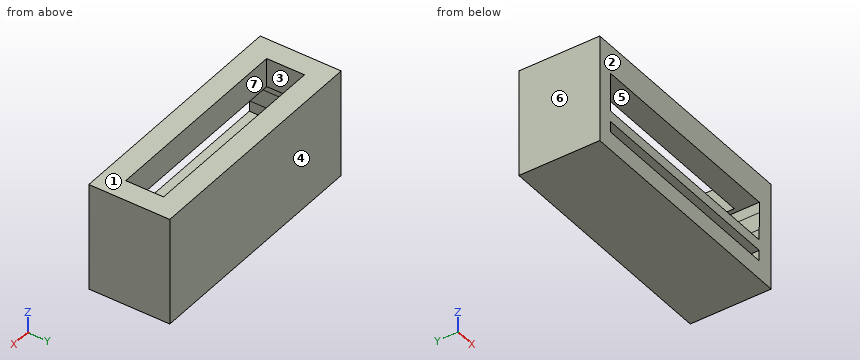
```python
from build123d import *

# Parameters (mm, degrees)
F0_W     = 114.3
F0_H     = 38.1
F1_DEPTH = 50.8
F2_W     = 93.98
F2_H     = 17.78
F3_DEPTH = 38.1
F4_W     = 99.06
F4_H     = 5.08
F5_DEPTH = 25.4
F6_DEPTH = 25.4


# Not quite as in the source:
# - a feature names something its author has since deleted; it is built from what else it names


with BuildPart() as f1:
    # F0 (on Top) → F1 (new body)
    with BuildSketch(Plane.XY):
        with Locations((-0.8744271472, -29.0754930802)):
            Rectangle(F0_W, F0_H)
    extrude(amount=F1_DEPTH)

    # F2 (on face) → F3 (cut)
    with BuildSketch(Plane.XY.offset(50.8)):
        with Locations((-0.8926133716, -29.0383800721)):
            Rectangle(F2_W, F2_H)
    extrude(amount=-F3_DEPTH, mode=Mode.SUBTRACT)

    # F4 (on face) → F5 (cut)
    with BuildSketch(Plane.XZ.offset(48.1254930802)):
        with Locations((-1.2216676867, 11.2467280274)):
            Rectangle(F4_W, F4_H)
        Polygon((-50.7150366902, 32.0992726219), (-50.7516676867, 23.9467280274), (48.3083323133, 23.9467280274), (48.3449633098, 32.0992726219), align=None)
        with Locations((-1.2216676867, 21.4067280274)):
            Rectangle(F4_W, F4_H)
        with Locations((-1.1850366902, 34.6392726219)):
            Rectangle(F4_W, F4_H)
    extrude(amount=-F5_DEPTH, mode=Mode.SUBTRACT)

    # F4 (on face) → F6 (cut)
    with BuildSketch(Plane.XZ.offset(48.1254930802)):
        with Locations((-1.2216676867, 11.2467280274)):
            Rectangle(F4_W, F4_H)
        Polygon((-50.7150366902, 32.0992726219), (-50.7516676867, 23.9467280274), (48.3083323133, 23.9467280274), (48.3449633098, 32.0992726219), align=None)
        with Locations((-1.2216676867, 21.4067280274)):
            Rectangle(F4_W, F4_H)
        with Locations((-1.1850366902, 34.6392726219)):
            Rectangle(F4_W, F4_H)
    extrude(amount=-F6_DEPTH, mode=Mode.SUBTRACT)


solid = f1.part
```
Read the model definition and answer for the solid it produces. Units are mm, in the model's axes. Face numbers are marked on the shaded views. A direction names the side the tool comes from. Coordinates: 2 decimals unless noted, no trailing zeros. Write each loop counter-clockwise with the first axis right and the second up, starting at its lowest first coordinate (ties: lowest second). Pieces come first, ordered by that corner, then holes. Notation, with made-up numbers: (49, 55) - (67, 55) arc R6 ccw to (67, 64) - close; hole circle Ø10 at (-15, -15.75). An arc over 180 degrees is marked (long way). Answer as a JSON object with one key per item and string values. Group by question number.
1. Which of the six approach directions +Z, -Z, +X, -X, +Y, -Y give full straight-line access (tool end or side, diameter ignored) to the marked faces 5, 6 and 7?
2. A cutting plane is placed at C-C (x = -32). Determine the outline of the cut face in (y, z), plus the area to 3 significant figures.
3. The mould has two halves that part along Y. Classify the marked faces 1, 2, 3 and 4: +Y half, -Y half, draft (parallel to the pull), parting line (faces both ways), or undercut.
4. Consider L1, parallel to Z at x = 14, y = -41; L2, parallel to X at y = -29, z = 49.5; L3, parallel to X at y = -28.5, z = 37. Determine where each line is inside the solid, lowest interval first. Write a range as [from, to].
5. Each of these flat-tipped pins is pushed along its axis until it touches: P1, Ø1.3, axis at x = 8, y = -21, coming from the +Z side; P2, Ø2.5, axis at x = -26, z = 12, coming from the -Y side; P3, Ø12.5, axis at x = -22.5, y = -29.5, coming from the +Z side. Where does it stop, or does it pass through?
6. A cutting plane is placed at B-B (y = -43.5). Determine the outline of the cut face in (x, z).
7. A cutting plane is placed at A-A (z = 42). Determine the outline of the cut face in (x, y).
8. A cutting plane is placed at D-D (y = -24.5). Determine the outline of the cut face in (x, z).
Worked out:
{
 "1": {"face 5": "-Y", "face 6": "+Z, -Z, -X, +Y, -Y", "face 7": "+Z"},
 "2": {"outline": "(-48.13, 0) - (-10.03, 0) - (-10.03, 50.8) - (-20.15, 50.8) - (-20.15, 12.7) - (-22.73, 12.7) - (-22.73, 8.71) - (-48.13, 8.71) - close; (-48.13, 13.79) - (-37.93, 13.79) - (-37.93, 18.87) - (-48.13, 18.87) - close; (-48.13, 37.18) - (-37.93, 37.18) - (-37.93, 50.8) - (-48.13, 50.8) - close", "area": "959 mm²"},
 "3": {"face 1": "draft", "face 2": "-Y half", "face 3": "undercut", "face 4": "+Y half"},
 "4": {"L1": "z = [0, 8.71], [13.79, 18.87], [37.18, 50.8]", "L2": "x = [-58.02, -47.88], [46.1, 56.28]", "L3": "x = [-58.02, -50.72], [48.34, 56.28]"},
 "5": {"P1": "stops at z = 12.7", "P2": "stops at y = -22.73", "P3": "stops at z = 8.71"},
 "6": {"outline": "(-58.02, 0) - (56.28, 0) - (56.28, 50.8) - (-58.02, 50.8) - close; hole (-50.75, 8.71) - (48.31, 8.71) - (48.31, 13.79) - (-50.75, 13.79) - close; hole (-50.75, 18.87) - (48.31, 18.87) - (48.31, 23.95) - (48.34, 32.1) - (48.34, 37.18) - (-50.72, 37.18) - (-50.72, 32.1) - (-50.75, 23.95) - close"},
 "7": {"outline": "(-58.02, -48.13) - (56.28, -48.13) - (56.28, -10.03) - (-58.02, -10.03) - close; hole (-47.88, -37.93) - (46.1, -37.93) - (46.1, -20.15) - (-47.88, -20.15) - close"},
 "8": {"outline": "(-58.02, 0) - (56.28, 0) - (56.28, 50.8) - (46.1, 50.8) - (46.1, 37.18) - (48.34, 37.18) - (48.34, 32.1) - (48.31, 23.95) - (48.31, 18.87) - (46.1, 18.87) - (46.1, 13.79) - (48.31, 13.79) - (48.31, 8.71) - (-50.75, 8.71) - (-50.75, 13.79) - (-47.88, 13.79) - (-47.88, 18.87) - (-50.75, 18.87) - (-50.75, 23.95) - (-50.72, 32.1) - (-50.72, 37.18) - (-47.88, 37.18) - (-47.88, 50.8) - (-58.02, 50.8) - close"}
}
